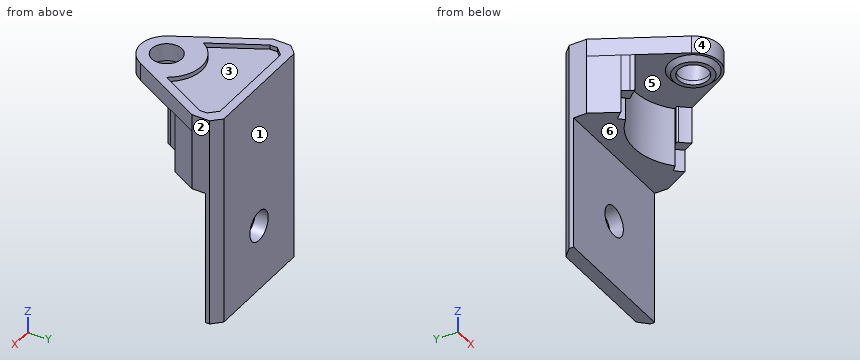
from build123d import *
from build123d.topology import SkipClean

# Parameters (mm, degrees)
BOSS_EXTRUDE1_DEPTH  = 2
BOSS_EXTRUDE2_START  = 4.75
BOSS_EXTRUDE2_DEPTH  = 4.75
BOSS_EXTRUDE3_START  = 2
SKETCH3_R            = 3
SKETCH3_R_2          = 1.7
BOSS_EXTRUDE3_DEPTH  = 2
SKETCH4_R            = 2.2
SKETCH4_R_2          = 1.7
BOSS_EXTRUDE4_DEPTH  = 0.5
CHAMFER1_SIZE        = 0.5
SKETCH5_W            = 7.5
SKETCH5_H            = 3
BOSS_EXTRUDE5_DEPTH  = 2
BOSS_EXTRUDE6_DEPTH  = 4.2
BOSS_EXTRUDE8_DEPTH  = 6.75
SKETCH10_W           = 15
SKETCH10_H           = 3
BOSS_EXTRUDE9_DEPTH  = 15.25
SKETCH11_R           = 1.65
CUT_EXTRUDE1_DEPTH   = 22.542109925
FILLET1_R            = 0.2
CHAMFER6_SIZE        = 1.5
BOSS_EXTRUDE12_REACH = 29.249
SKETCH16_W           = 15
SKETCH16_H           = 1.5
CUT_EXTRUDE3_DEPTH   = 0.5
CHAMFER7_SIZE        = 1
CUT_EXTRUDE4_DEPTH   = 15.25
SKETCH18_R           = 1.7
CUT_EXTRUDE5_DEPTH   = 10


with BuildPart() as part:
    # Sketch1 → Boss-Extrude1 (new body)
    with BuildSketch(Plane.XY):
        with BuildLine():
            Line((4.594082841, 4.876925553), (5.159993549, 5.442836262))
            ThreePointArc((5.159993549, 5.442836262), (0, 7.5), (-5.159993549, 5.442836262))
            Line((-5.159993549, 5.442836262), (-4.594082841, 4.876925553))
            ThreePointArc((-4.594082841, 4.876925553), (0, 6.7), (4.594082841, 4.876925553))
        make_face()
    extrude(amount=-BOSS_EXTRUDE1_DEPTH)

    # Sketch1<3> → Boss-Extrude2 (add)
    with BuildSketch(Plane.XY.offset(BOSS_EXTRUDE2_START)):
        with BuildLine():
            Line((4.594082841, 4.876925553), (5.159993549, 5.442836262))
            ThreePointArc((5.159993549, 5.442836262), (0, 7.5), (-5.159993549, 5.442836262))
            Line((-5.159993549, 5.442836262), (-4.594082841, 4.876925553))
            ThreePointArc((-4.594082841, 4.876925553), (0, 6.7), (4.594082841, 4.876925553))
        make_face()
    extrude(amount=-BOSS_EXTRUDE2_DEPTH)

    # Sketch3 → Boss-Extrude3 (add)
    # profile 1 of 4: a face of its own
    with BuildSketch(Plane.XY.offset(4.75).offset(BOSS_EXTRUDE3_START)):
        with BuildLine():
            Line((-4.594082841, 4.876925553), (-5.159993549, 5.442836262))
            Line((-5.159993549, 5.442836262), (-2.820975701, -1.02083108))
            ThreePointArc((-2.820975701, -1.02083108), (-2.892694114, 0.795185994), (-1.902774006, 2.31936437))
            Line((-1.902774006, 2.31936437), (-2.780654635, 4.745309242))
            ThreePointArc((-2.780654635, 4.745309242), (0, 5.5), (2.780654635, 4.745309242))
            Line((2.780654635, 4.745309242), (1.902774006, 2.31936437))
            ThreePointArc((1.902774006, 2.31936437), (2.711855639, 1.282902565), (3, 0))
            ThreePointArc((3, 0), (2.954904999, -0.518205025), (2.820975701, -1.02083108))
            Line((2.820975701, -1.02083108), (5.159993549, 5.442836262))
            Line((5.159993549, 5.442836262), (4.594082841, 4.876925553))
            ThreePointArc((4.594082841, 4.876925553), (0, 6.7), (-4.594082841, 4.876925553))
        make_face()
    # profile 2 of 4: a face of its own
    with BuildSketch(Plane.XY.offset(4.75).offset(BOSS_EXTRUDE3_START)):
        with BuildLine():
            Line((-5.159993549, 5.442836262), (-4.594082841, 4.876925553))
            ThreePointArc((-4.594082841, 4.876925553), (0, 6.7), (4.594082841, 4.876925553))
            Line((4.594082841, 4.876925553), (5.159993549, 5.442836262))
            ThreePointArc((5.159993549, 5.442836262), (0, 7.5), (-5.159993549, 5.442836262))
        make_face()
    # profile 3 of 4: a face of its own
    with BuildSketch(Plane.XY.offset(4.75).offset(BOSS_EXTRUDE3_START)):
        Circle(SKETCH3_R)
        Circle(SKETCH3_R_2, mode=Mode.SUBTRACT)
    # profile 4 of 4: a face of its own
    with BuildSketch(Plane.XY.offset(4.75).offset(BOSS_EXTRUDE3_START)):
        with BuildLine():
            Line((-2.780654635, 4.745309242), (-1.902774006, 2.31936437))
            ThreePointArc((-1.902774006, 2.31936437), (0, 3), (1.902774006, 2.31936437))
            Line((1.902774006, 2.31936437), (2.780654635, 4.745309242))
            ThreePointArc((2.780654635, 4.745309242), (0, 5.5), (-2.780654635, 4.745309242))
        make_face()
    extrude(amount=-BOSS_EXTRUDE3_DEPTH)

    # Sketch4 → Boss-Extrude4 (add)
    with SkipClean():  # the faces are left unmerged after this step: merging them gives an invalid solid
        with BuildSketch(Plane(origin=(0, 0, 4.75), x_dir=(-1, 0, 0), z_dir=(0, 0, -1))):
            with Locations(Location((0, 0, 0), (0, 0, 180))):
                Circle(SKETCH4_R)
            Circle(SKETCH4_R_2, mode=Mode.SUBTRACT)
        extrude(amount=BOSS_EXTRUDE4_DEPTH)
    add(part.part.scale(1), mode=Mode.REPLACE)  # the faces are merged on a copy

    # Chamfer1
    chamfer1_edges = [part.edges().sort_by_distance(p)[0] for p in [
        (-2.2, 0, 4.75),
    ]]
    chamfer(chamfer1_edges, length=CHAMFER1_SIZE - 0.0001)  # a hair under: the kernel refuses the full size

    # Sketch5 → Boss-Extrude5 (add)
    with BuildSketch(Plane.XY.offset(6.75)):
        with BuildLine():
            ThreePointArc((-5.159993549, 5.442836262), (-2.777474396, 6.966752183), (0, 7.5))
            Line((0, 7.5), (-7.5, 7.5))
            Line((-7.5, 7.5), (-2.634698995, -1.434698995))
            ThreePointArc((-2.634698995, -1.434698995), (-2.735675101, -1.231292711), (-2.820975701, -1.02083108))
            Line((-2.820975701, -1.02083108), (-5.159993549, 5.442836262))
        make_face()
        with Locations((-3.75, 9)):
            Rectangle(SKETCH5_W, SKETCH5_H)
        with Locations((3.75, 9)):
            Rectangle(SKETCH5_W, SKETCH5_H)
        with BuildLine():
            Line((7.5, 7.5), (0, 7.5))
            ThreePointArc((0, 7.5), (2.777474396, 6.966752183), (5.159993549, 5.442836262))
            Line((5.159993549, 5.442836262), (2.820975701, -1.02083108))
            ThreePointArc((2.820975701, -1.02083108), (2.756369418, -1.184241374), (2.682306676, -1.343588812))
            Line((2.682306676, -1.343588812), (7.5, 7.5))
        make_face()
    extrude(amount=-BOSS_EXTRUDE5_DEPTH)

    # Sketch6 → Boss-Extrude6 (add)
    with SkipClean():  # the faces are left unmerged after this step: merging them gives an invalid solid
        with BuildSketch(Plane(origin=(0, 0, 4.75), x_dir=(-1, 0, 0), z_dir=(0, 0, -1))):
            with BuildLine():
                Line((-5.921621025, 4.602651891), (-5.499242594, 3.827313795))
                ThreePointArc((-5.499242594, 3.827313795), (-5.073876801, 4.375588441), (-4.594082841, 4.876925553))
                Line((-4.594082841, 4.876925553), (-5.159993549, 5.442836262))
                ThreePointArc((-5.159993549, 5.442836262), (-5.556709713, 5.037159632), (-5.921621025, 4.602651891))
            make_face()
            with BuildLine():
                Line((5.159993549, 5.442836262), (4.594082841, 4.876925553))
                ThreePointArc((4.594082841, 4.876925553), (5.074143899, 4.375278699), (5.499709828, 3.826642367))
                Line((5.499709828, 3.826642367), (5.922007367, 4.602154794))
                ThreePointArc((5.922007367, 4.602154794), (5.556921127, 5.036926403), (5.159993549, 5.442836262))
            make_face()
            with BuildLine():
                Line((-5.499242594, 3.827313795), (-5.256310338, 3.381375701))
                ThreePointArc((-5.256310338, 3.381375701), (-4.806527723, 3.994970744), (-4.285525038, 4.549370852))
                Line((-4.285525038, 4.549370852), (-4.594082841, 4.876925553))
                ThreePointArc((-4.594082841, 4.876925553), (-5.073876801, 4.375588441), (-5.499242594, 3.827313795))
            make_face()
            with BuildLine():
                Line((4.594082841, 4.876925553), (4.275732705, 4.558575417))
                ThreePointArc((4.275732705, 4.558575417), (4.802528974, 3.999776925), (5.256816116, 3.380589346))
                Line((5.256816116, 3.380589346), (5.499709828, 3.826642367))
                ThreePointArc((5.499709828, 3.826642367), (5.074143899, 4.375278699), (4.594082841, 4.876925553))
            make_face()
        extrude(amount=BOSS_EXTRUDE6_DEPTH)

    # Sketch8 → Boss-Extrude8 (add)
    with BuildSketch(Plane(origin=(0, 0, 4.75), x_dir=(-1, 0, 0), z_dir=(0, 0, -1))):
        with BuildLine():
            Line((5.922007367, 4.602154794), (7.5, 7.5))
            Line((7.5, 7.5), (7.5, 10.5))
            Line((7.5, 10.5), (-7.5, 10.5))
            Line((-7.5, 10.5), (-7.5, 7.5))
            Line((-7.5, 7.5), (-5.921621025, 4.602651891))
            ThreePointArc((-5.921621025, 4.602651891), (0.000314788, 7.499999993), (5.922007367, 4.602154794))
        make_face()
    extrude(amount=BOSS_EXTRUDE8_DEPTH)

    # Sketch10 → Boss-Extrude9 (add)
    with BuildSketch(Plane(origin=(0, 0, -2), x_dir=(-1, 0, 0), z_dir=(0, 0, -1))):
        with Locations((0, 9)):
            Rectangle(SKETCH10_W, SKETCH10_H)
    extrude(amount=BOSS_EXTRUDE9_DEPTH)

    # Sketch11 → Cut-Extrude1 (cut, through all)
    with BuildSketch(Plane.XZ.offset(-7.5)):
        with Locations(Location((0, -9.5, 0), (0, 0, 270))):
            Circle(SKETCH11_R)
    extrude(amount=-CUT_EXTRUDE1_DEPTH, mode=Mode.SUBTRACT)

    # Fillet1
    fillet1_edges = [part.edges().sort_by_distance(p)[0] for p in [
        (4.285525038, 4.549370852, 2.65),
        (-4.275732705, 4.558575417, 2.65),
    ]]
    fillet(fillet1_edges, radius=FILLET1_R)

    # Chamfer6
    chamfer6_edges = [part.edges().sort_by_distance(p)[0] for p in [
        (7.5, 10.5, -5.25),
        (-7.5, 10.5, -5.25),
    ]]
    chamfer(chamfer6_edges, length=CHAMFER6_SIZE)

    # Boss-Extrude12: up to this face of the body (flat: up to its plane)
    boss_extrude12_end = Plane(part.part.faces().sort_by_distance((-0.00029363, 5.45528482, 6.75))[0])
    # Sketch16 → Boss-Extrude12 (add, up to the picked face)
    with BuildSketch(Plane(origin=(0, 0, -17.25), x_dir=(-1, 0, 0), z_dir=(0, 0, -1)), mode=Mode.PRIVATE) as boss_extrude12_sk1:
        with Locations((0, 9.75)):
            Rectangle(SKETCH16_W, SKETCH16_H)
    boss_extrude12_tool1 = split(extrude(boss_extrude12_sk1.sketch, amount=-BOSS_EXTRUDE12_REACH, mode=Mode.PRIVATE), bisect_by=boss_extrude12_end, keep=Keep.BOTH, mode=Mode.PRIVATE)
    add(boss_extrude12_tool1.solids().sort_by(Axis((0, 9.75, -17.25), (0, 0, 1)))[0])

    # Sketch13 → Cut-Extrude3 (cut)
    with BuildSketch(Plane.XY.offset(6.75)):
        with BuildLine():
            ThreePointArc((3.4124071, 2.086978147), (-0.000677338, 3.999999943), (-3.413113698, 2.085822351))
            Line((-3.413113698, 2.085822351), (-6.5, 7.754618569))
            Line((-6.5, 7.754618569), (-6.5, 8.585786438))
            Line((-6.5, 8.585786438), (-5.585786438, 9.5))
            Line((-5.585786438, 9.5), (5.585786438, 9.5))
            Line((5.585786438, 9.5), (6.5, 8.585786438))
            Line((6.5, 8.585786438), (6.5, 7.754711685))
            Line((6.5, 7.754711685), (3.4124071, 2.086978147))
        make_face()
    extrude(amount=-CUT_EXTRUDE3_DEPTH, mode=Mode.SUBTRACT)

    # Chamfer7
    chamfer7_edges = [part.edges().sort_by_distance(p)[0] for p in [
        (7.5, 10.5, -5.25),
        (-7.5, 10.5, -5.25),
    ]]
    chamfer(chamfer7_edges, length=CHAMFER7_SIZE)

    # Sketch17 → Cut-Extrude4 (cut)
    with BuildSketch(Plane(origin=(0, 0, -17.25), x_dir=(-1, 0, 0), z_dir=(0, 0, -1))):
        Polygon((7.5, 9), (-6.884093455, 9), (-7.5, 9), (-7.5, 7.5), (7.5, 7.5), align=None)
    extrude(amount=-CUT_EXTRUDE4_DEPTH, mode=Mode.SUBTRACT)

    # Sketch18 → Cut-Extrude5 (cut)
    with BuildSketch(Plane(origin=(0, 10.5, 0), x_dir=(1, 0, 0), z_dir=(0, 1, 0))):
        with Locations(Location((0, 9.75, 0), (0, 0, 180))):
            Circle(SKETCH18_R)
    extrude(amount=-CUT_EXTRUDE5_DEPTH, mode=Mode.SUBTRACT)


solid = part.part
Design review of the part built by this model. Coordinates are the model's own, in mm. Face numbers are marked on the shaded views. A direction names the side the tool comes from. Coordinates: 2 decimals unless noted, no trailing zeros. Write each loop counter-clockwise with the first axis right and the second up, starting at its lowest first coordinate (ties: lowest second). Pieces come first, ordered by that corner, then holes. Notation, with made-up numbers: (-37.5, 0) - (-16.5, 0) arc R14 cw to (-16.5, 16) - close; hole circle Ø8 at (12, 54.25). An arc over 180 degrees is marked (long way). Use one line per item in the form item = value.
Q1. Insertion check: pin 1 Ø1.2 at (x, y) = (5.5, 4.5) entering from -Z; pin 2 Ø1.5 at (x, y) = (4, 0) entering from -Z; pin 3 Ø0.5 at (x, y) = (-5, 4.5) entering from -Z; pin 4 Ø1.3 at (x, y) = (-0.5, -0.5) entering from -Z. Each pin has a flat end and moves straight along its axis. Give the tip position at first contact, or say it passes through.
Taken from the geometry:
pin_1 = -2
pin_2 = 4.75
pin_3 = 0.55
pin_4 = through
Q2. Consider section A-A (x = 0). Count the separate pieces of the cut face and the enclosed holes in it, plus the area to 3 significant figures.
Taken from the geometry:
separate_pieces = 3
enclosed_holes = 0
area = 61.6 mm^2
Q3. Consider section D-D (y = 5.75). Write out the cut boundary in (x, z).
Taken from the geometry:
outline = (-6.55, -2) - (-3.44, -2) - (-3.44, 4.75) - (3.44, 4.75) - (3.44, -2) - (6.55, -2) - (6.55, 6.75) - (5.41, 6.75) - (5.41, 6.25) - (-5.41, 6.25) - (-5.41, 6.75) - (-6.55, 6.75) - close
Q4. Consider section B-B (z = -8.5). Write out the cut boundary in (x, y), plus the area to 3 significant figures.
Taken from the geometry:
outline = (-7.5, 9) - (-1.15, 9) - (-1.15, 10.5) - (-6.5, 10.5) - (-7.5, 9.5) - close; (1.15, 9) - (7.5, 9) - (7.5, 9.5) - (6.5, 10.5) - (1.15, 10.5) - close
area = 18.0 mm^2
Q5. The part is to be moulded in two halves that separate along Y. For the marked faces 1, 2 and 3, say which applies: +Y half, -Y half, draft (parallel to the pull), parting line (faces both ways), or undercut.
Taken from the geometry:
face_1 = +Y half
face_2 = draft
face_3 = undercut
Q6. For probe 1 along Y at (x, z) = (0, 6.35); probe 2 along Y at (x, z) = (0, 5.25); probe 3 along Z at (x, y) = (0, 9.95), list the stretches that pass through material, from the lowest coordinate up.
Taken from the geometry:
probe_1 = -3 to -1.7, 1.7 to 4, 9.5 to 10.5
probe_2 = -3 to -1.7, 1.7 to 10.5
probe_3 = -17.25 to -11.45, -8.05 to 6.75
Q7. Machinability: for the marked faces 4, 5 and 6, which of the approach directions +Z, -Z, +X, -X, +Y, -Y give a long, thin tool a straight path to every point of the face, cutting with its end or side? Answer none if there is none.
Taken from the geometry:
face_4 = +Z, -Z, -Y
face_5 = -Z
face_6 = -Z, +X, -X, -Y
